Study the drawing (mm; zero at the part's minimum x, y, z) and answer. A direction names the side the tool comes from. Coordinates: 2 decimals unless noted, no trailing zeros. Order: outer loops, then holes, each group sorted by start corner. A loop starts at its lowest first (then second) coordinate and runs counter-clockwise, first axis right, second up.
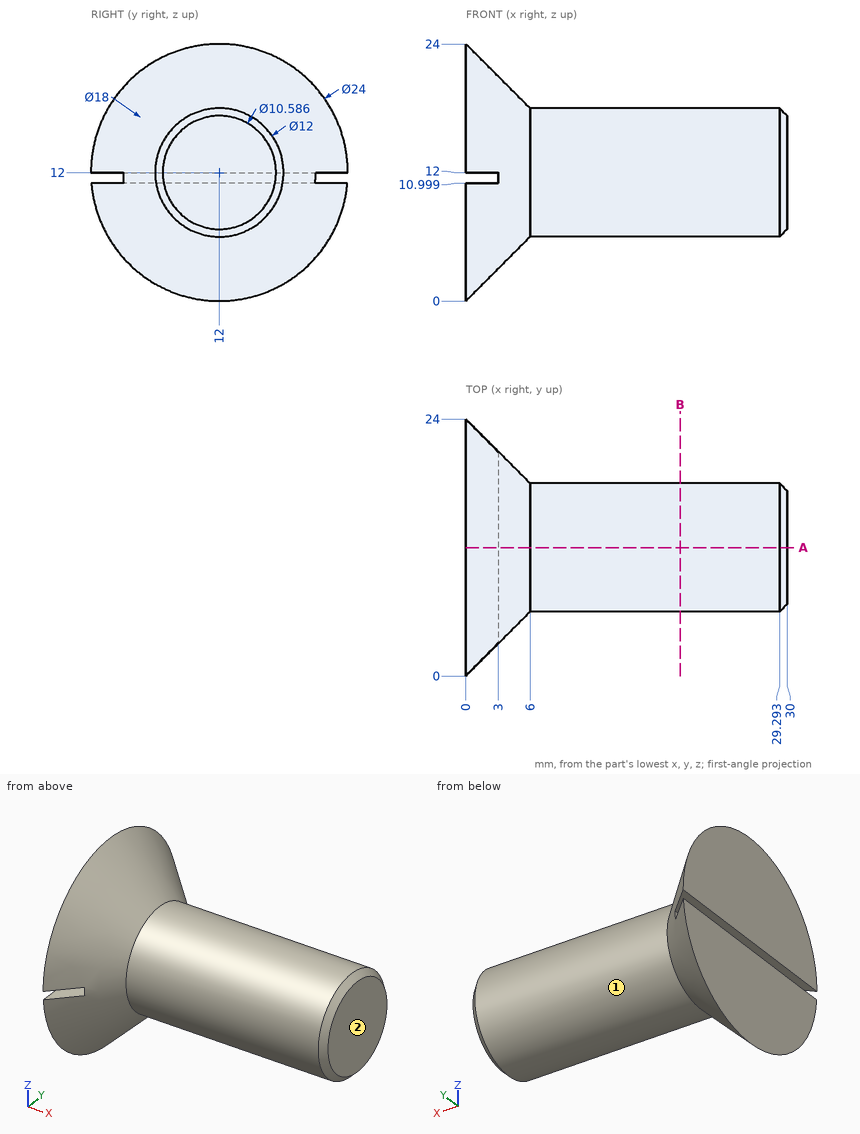
1) Which of the six approach directions +Z, -Z, +X, -X, +Y, -Y give full straight-line access (tool end or side, diameter ignored) to the marked faces 1 and 2?
A:
face 1: +X
face 2: +Z, -Z, +X, +Y, -Y
2) Flat-ended cylindrical pins translate along their axes: pin 1 Ø6 at (x, z) = (11, 14.5) entering from -Y; pin 2 Ø12 at (x, z) = (6, 20) entering from +Y; pin 3 Ø1 at (x, y) = (8, 18) entering from -Z. Find the tip coordinate at first contact, or state that the pin passes through.
A:
pin 1: stops at y = 6
pin 2: stops at y = 22.05
pin 3: stops at z = 9.6
3) A cutting plane is placed at A-A, the plane y = 12. Determine the outline of the cut face in (x, z), and give its area (4 significant figures).
A:
outline: (0, 0) - (6, 6) - (29.29, 6) - (30, 6.71) - (30, 17.29) - (29.29, 18) - (6, 18) - (0, 24) - (0, 12) - (3, 12) - (3, 11) - (0, 11) - close
area: 392.5 mm2
4) Straight lines are drawn through the part: line 1 (Z direction, x = 2.5, y = 15) (1 decimal); line 2 (X direction, y = 13, z = 6.25); line 3 (Y direction, x = 26, z = 15.5). For each, find the intervals that lie inside material, in ascending order.
A:
line 1: z = 3 to 11, 12 to 21
line 2: x = 0 to 29.46
line 3: y = 7.13 to 16.87
5) A cutting plane is placed at B-B, the plane x = 20. Determine the outline of the cut face in (y, z).
A:
outline: circle Ø12 at (12, 12)
